```python
from build123d import *

# Parameters (mm, degrees)
SKETCH1_W           = 34.539950858
SKETCH1_H           = 14.819505943
SKETCH1_W_2         = 42.327470122
SKETCH1_H_2         = 10
BOSS_EXTRUDE1_DEPTH = 3


with BuildPart() as part:
    # Sketch1 → Boss-Extrude1 (new body)
    with BuildSketch(Plane.XY):
        Polygon((0, 0), (0, 5), (-3, 5), (-3, 15), (0, 15), (0, 20), (30, 20), (30, 23), (90, 23), (90, 20), (120, 20), (120, 15), (123, 15), (123, 5), (120, 5), (120, 0), (90, 0), (90, -3), (30, -3), (30, 0), align=None)
        with Locations((29.364361229, 11.580788204)):
            Rectangle(SKETCH1_W, SKETCH1_H, mode=Mode.SUBTRACT)
        with Locations((70.779364133, 10)):
            Rectangle(SKETCH1_W_2, SKETCH1_H_2, mode=Mode.SUBTRACT)
    extrude(amount=BOSS_EXTRUDE1_DEPTH)


solid = part.part
```
Input: part model. Units: mm. Frame: model coordinates. A direction names the side the tool comes from. Coordinates: 2 decimals unless noted, no trailing zeros. Loops run counter-clockwise (first coordinate to the right, second up) from the corner with the lowest first, then second, coordinate; pieces in that order, holes last. Notation, with made-up numbers: M 66.5,32 L 124.5,32 A17 cw 124.5,51 Z; hole C -0.75,50.5 d8. An arc over 180 degrees is marked long. Use a Markdown table: item, result. Add a question column.
1) Section B-B, the plane y = 10. Return the cut outline in (x, z), plus the area to 3 significant figures.
2) Pin query (flat end, axial travel): P1, Ø0.9, axis at x = 19, z = 1, coming from the +Y side; P2, Ø1.5, axis at x = 121.5, z = 1.5, coming from the +Y side; P3, Ø6, axis at x = 61, y = 10.5, coming from the -Z side; P4, Ø1.5, axis at y = -1.5, z = 1.5, coming from the +X side. Return the tip coordinate at first contact, or that it passes through.
3) Draft query along X for faces 4 (the flat face through (60, -3, 1)), 5 (the flat face through (30, -2, 1)), 6 (the flat face through (12.094, 11, 1)), 7 (the flat face through (120, 18, 1)). Return one class per face: +X half, -X half, draft (parallel to the pull), parting line (faces both ways), or undercut.
4) Section D-D, the plane y = 16.25. Return the cut outline in (x, z), plus the area to 3 significant figures.
5) Section C-C, the plane z = 1.45. Return the cut outline in (x, y), plus the area to 3 significant figures.
6) Section A-A, the plane x = 36. Return the cut outline in (y, z).
7) Set-up query: faces 1 (the flat face through (-2, 15, 1)), 2 (the flat face through (70, 15, 1)), 3 (the flat face through (-1, 5, 1)). Return all of +Z, -Z, +X, -X, +Y, -Y with unobstructed straight access to the full face (end or side cutting, diameter ignored); none if empty.
8) Line query: L1, parallel to X at y = 8.5, z = 1.85; L2, parallel to Y at x = 36, z = 2.55; L3, parallel to Y at x = 16, z = 0.7. Output: solid intervals per line, ascending. Write a range as from..to.
Answer below:
| question | item | result |
|---|---|---|
| 1 | outline | M -3,0 L 12.09,0 L 12.09,3 L -3,3 Z; M 46.63,0 L 49.62,0 L 49.62,3 L 46.63,3 Z; M 91.94,0 L 123,0 L 123,3 L 91.94,3 Z |
| 1 | area | 147 mm2 |
| 2 | P1 | y = 20 |
| 2 | P2 | y = 15 |
| 2 | P3 | through |
| 2 | P4 | x = 90 |
| 3 | face 4 | draft |
| 3 | face 5 | -X half |
| 3 | face 6 | undercut |
| 3 | face 7 | +X half |
| 4 | outline | M 0,0 L 12.09,0 L 12.09,3 L 0,3 Z; M 46.63,0 L 120,0 L 120,3 L 46.63,3 Z |
| 4 | area | 256 mm2 |
| 5 | outline | M -3,5 L 0,5 L 0,0 L 30,0 L 30,-3 L 90,-3 L 90,0 L 120,0 L 120,5 L 123,5 L 123,15 L 120,15 L 120,20 L 90,20 L 90,23 L 30,23 L 30,20 L 0,20 L 0,15 L -3,15 Z; hole M 12.09,4.17 L 46.63,4.17 L 46.63,18.99 L 12.09,18.99 Z; hole M 49.62,5 L 91.94,5 L 91.94,15 L 49.62,15 Z |
| 5 | area | 1,880 mm2 |
| 6 | outline | M -3,0 L 4.17,0 L 4.17,3 L -3,3 Z; M 18.99,0 L 23,0 L 23,3 L 18.99,3 Z |
| 7 | face 1 | +Z, -Z, -X, +Y |
| 7 | face 2 | +Z, -Z |
| 7 | face 3 | +Z, -Z, -X, -Y |
| 8 | L1 | -3..12.09, 46.63..49.62, 91.94..123 |
| 8 | L2 | -3..4.17, 18.99..23 |
| 8 | L3 | 0..4.17, 18.99..20 |
